from build123d import *

# Parameters (mm, degrees)
BOSS_EXTRUDE1_DEPTH  = 3.15
SKETCH3_W            = 12.18
SKETCH3_H            = 10.02
SKETCH3_W_2          = 8.18
SKETCH3_H_2          = 5.02
BOSS_EXTRUDE2_DEPTH  = 1.5
SKETCH5_W            = 12.18
SKETCH5_H            = 10.02
CUT_EXTRUDE1_DEPTH   = 0.3
SKETCH7_W            = 50
SKETCH7_H            = 80
SKETCH7_W_2          = 12.18
SKETCH7_H_2          = 10.02
BOSS_EXTRUDE7_DEPTH  = 2.85
SKETCH8_W            = 50
SKETCH8_H            = 20
BOSS_EXTRUDE8_DEPTH  = 10
SKETCH9_W            = 18.91
SKETCH9_H            = 6.02
CUT_EXTRUDE2_DEPTH   = 1.35
SKETCH11_W           = 20
SKETCH11_H           = 16.49
BOSS_EXTRUDE9_DEPTH  = 8.5
BOSS_EXTRUDE10_DEPTH = 8.1
CUT_EXTRUDE3_DEPTH   = 10


with BuildPart() as part:
    # Sketch1 → Boss-Extrude1 (new body)
    with BuildSketch(Plane(origin=(0, 0, 0), x_dir=(1, 0, 0), z_dir=(0, 1, 0))):
        Polygon((-0.5, -0.5), (8.68, -0.5), (8.68, 0), (10.18, 0), (10.18, -2), (-2, -2), (-2, 8.02), (10.18, 8.02), (10.18, 6.02), (8.68, 6.02), (8.68, 6.52), (-0.5, 6.52), align=None)
    extrude(amount=BOSS_EXTRUDE1_DEPTH)

    # Sketch3 → Boss-Extrude2 (add)
    with BuildSketch(Plane(origin=(0, 3.15, 0), x_dir=(1, 0, 0), z_dir=(0, 1, 0))):
        with Locations((4.09, 3.01)):
            Rectangle(SKETCH3_W, SKETCH3_H)
        with Locations((4.59, 3.01)):
            Rectangle(SKETCH3_W_2, SKETCH3_H_2, mode=Mode.SUBTRACT)
    extrude(amount=-BOSS_EXTRUDE2_DEPTH)

    # Sketch5 → Cut-Extrude1 (cut)
    with BuildSketch(Plane.XZ):
        with Locations((4.09, -3.01)):
            Rectangle(SKETCH5_W, SKETCH5_H)
    extrude(amount=-CUT_EXTRUDE1_DEPTH, mode=Mode.SUBTRACT)

    # Sketch7 → Boss-Extrude7 (add)
    with BuildSketch(Plane(origin=(0, 3.15, 0), x_dir=(1, 0, 0), z_dir=(0, 1, 0))):
        with Locations((4.09, 3.01)):
            Rectangle(SKETCH7_W, SKETCH7_H)
        with Locations((4.09, 3.01)):
            Rectangle(SKETCH7_W_2, SKETCH7_H_2, mode=Mode.SUBTRACT)
    extrude(amount=-BOSS_EXTRUDE7_DEPTH)

    # Sketch8 → Boss-Extrude8 (add)
    with BuildSketch(Plane(origin=(0, 3.15, 0), x_dir=(1, 0, 0), z_dir=(0, 1, 0))):
        with Locations((4.09, -26.99)):
            Rectangle(SKETCH8_W, SKETCH8_H)
    boss_extrude8 = extrude(amount=BOSS_EXTRUDE8_DEPTH)

    # Sketch9 → Cut-Extrude2 (cut)
    with BuildSketch(Plane.XZ.offset(-0.3)):
        with Locations((19.635, -3.01)):
            Rectangle(SKETCH9_W, SKETCH9_H)
    extrude(amount=-CUT_EXTRUDE2_DEPTH, mode=Mode.SUBTRACT)

    # Sketch11 → Boss-Extrude9 (add)
    with BuildSketch(Plane(origin=(0, 3.15, 0), x_dir=(1, 0, 0), z_dir=(0, 1, 0))):
        with Locations((4.09, -8.745)):
            Rectangle(SKETCH11_W, SKETCH11_H)
    boss_extrude9 = extrude(amount=BOSS_EXTRUDE9_DEPTH)

    # Sketch12 → Boss-Extrude10 (add)
    with BuildSketch(Plane(origin=(0, 11.65, 0), x_dir=(1, 0, 0), z_dir=(0, 1, 0))):
        with BuildLine():
            Line((0, -0.5), (0, -16.99))
            Line((0, -16.99), (8.18, -16.99))
            Line((8.18, -16.99), (8.18, -0.5))
            ThreePointArc((8.18, -0.5), (4.09, -2.379638207), (0, -0.5))
        make_face()
    boss_extrude10 = extrude(amount=BOSS_EXTRUDE10_DEPTH)

    # Sketch13 → Cut-Extrude3 (cut)
    with BuildSketch(Plane(origin=(8.18, 0, 0), x_dir=(0, 0, -1), z_dir=(1, 0, 0))):
        Polygon((-16.99, 13.15), (-0.5, 19.75), (-16.99, 19.75), align=None)
    cut_extrude3 = extrude(amount=-CUT_EXTRUDE3_DEPTH, mode=Mode.SUBTRACT)

    # Mirror2: Boss-Extrude8, Boss-Extrude9, Boss-Extrude10, Cut-Extrude3 across plane
    add(boss_extrude8.mirror(Plane.XY.offset(-3.01)))
    add(boss_extrude9.mirror(Plane.XY.offset(-3.01)))
    add(boss_extrude10.mirror(Plane.XY.offset(-3.01)))
    add(cut_extrude3.mirror(Plane.XY.offset(-3.01)), mode=Mode.SUBTRACT)


solid = part.part
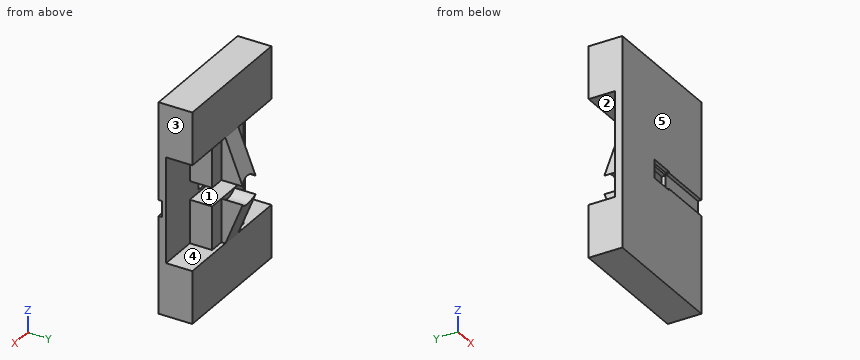
Work out the finished part from the listing and answer in its coordinate system (mm). Face numbers are marked on the shaded views. A direction names the side the tool comes from. Coordinates: 2 decimals unless noted, no trailing zeros. Loops run counter-clockwise (first coordinate to the right, second up) from the corner with the lowest first, then second, coordinate; pieces in that order, holes last. Notation, with made-up numbers: M -10,24 L 46,24 A37 ccw 46,62 Z; hole C 10.25,-4.75 d10. An arc over 180 degrees is marked long. Answer in a Markdown table with one row per item. Add a question column.
1. Find section B-B, the plane x = 12.5. Write down the section's boundary in (y, z).
2. Find section A-A, the plane y = 9. Write down the section's boundary in (x, z), then the cut area to 3 significant figures.
3. Consider L1, parallel to Z at x = 6, y = 3.25; L2, parallel to Z at x = -13.5, y = 3.75; L3, parallel to Y at x = -10.5, z = 10. Determine where each line is inside the solid, lowest interval first.
4. A tool of negligible diameter and unlimited length cuts with its end or side. For the marked faces 1, 2, 3, 4 and 5, from which of +Z, -Z, +X, -X, +Y, -Y can it reach the whole face along a straight path? Write none if from no direction.
5. Flat-ended cylindrical pins translate along their axes: P1, Ø5, axis at y = 17, z = 8.5, coming from the +X side; P2, Ø4, axis at y = 14, z = 10, coming from the -X side; P3, Ø0.9, axis at x = 3.5, z = 1.5, coming from the +Y side. Find the tip coordinate at first contact, or state that the pin passes through.
6. Find section D-D, the plane y = 15. Write down the section's boundary in (x, z), then the cut area to 3 significant figures.
7. Find section C-C, the plane z = 8. Write down the section's boundary in (x, y), then the cut area to 3 significant figures.
Reported:
| question | item | result |
|---|---|---|
| 1 | outline | M 0.3,-43.01 L 13.15,-43.01 L 13.15,-23.01 L 11.65,-23.01 L 11.65,-6.52 L 3.15,-6.52 L 3.15,0.5 L 11.65,0.5 L 11.65,16.99 L 13.15,16.99 L 13.15,36.99 L 0.3,36.99 L 0.3,0 L 1.65,0 L 1.65,-6.02 L 0.3,-6.02 Z |
| 2 | outline | M -20.91,-43.01 L 29.09,-43.01 L 29.09,-23.01 L 14.09,-23.01 L 14.09,-6.52 L -5.91,-6.52 L -5.91,-23.01 L -20.91,-23.01 Z; M -20.91,16.99 L -5.91,16.99 L -5.91,0.5 L 14.09,0.5 L 14.09,16.99 L 29.09,16.99 L 29.09,36.99 L -20.91,36.99 Z |
| 2 | area | 2,660 mm^2 |
| 3 | L1 | z = -43.01 to -6.52, 0.5 to 36.99 |
| 3 | L2 | z = -43.01 to -23.01, 16.99 to 36.99 |
| 3 | L3 | y = 0.3 to 3.15 |
| 4 | face 1 | +X, -X, +Y |
| 4 | face 2 | -X, +Y |
| 4 | face 3 | +Z, -Z, +X, +Y, -Y |
| 4 | face 4 | +X, +Y |
| 4 | face 5 | +Z, -Z, +X, -X, -Y |
| 5 | P1 | stops at x = 8.18 |
| 5 | P2 | stops at x = 0 |
| 5 | P3 | stops at y = 11.65 |
| 6 | outline | M 0,-18.39 L 8.18,-18.39 L 8.18,-6.52 A5.39 cw 0,-6.52 Z; M 0,0.5 A5.39 cw 8.18,0.5 L 8.18,12.37 L 0,12.37 Z |
| 6 | area | 173 mm^2 |
| 7 | outline | M -20.91,0.3 L 29.09,0.3 L 29.09,3.15 L 14.09,3.15 L 14.09,11.65 L 8.18,11.65 L 8.18,16.75 L 0,16.75 L 0,11.65 L -5.91,11.65 L -5.91,3.15 L -20.91,3.15 Z |
| 7 | area | 354 mm^2 |
